Here's how the part is built. I have some questions about the finished solid (model axes, mm). Round coordinates to 2 decimals unless told otherwise and drop trailing zeros. Write each loop counter-clockwise with the first axis right and the second up, starting at its lowest first coordinate (ties: lowest second). Pieces come first, ordered by that corner, then holes. Notation, with made-up numbers: (6, 43) -> (40, 43) arc R33 cw to (40, 80) -> close; hole circle Ø11 at (47.5, 9). An arc over 180 degrees is marked (long way). Put each result on its own line as item: value. Start each with the question number.
1) I want a section at A-A, the plane x = 6. List the corners of the cut face in (y, z) for me, then the cut area to 3 significant figures.
2) I want a section at B-B, the plane z = 8. List the corners of the cut face in (x, y) for me, then the cut area to 3 significant figures.
3) If I drill on line 1 along Z through (x, y) = (4.25, -94.5); line 2 along X through (y, z) = (-51.5, 18.5); line 3 along X through (y, z) = (-12.5, 24), over which ranges is the centre line in solid material (lowest first)? Write a range as [from, to].
4) Will these pins go through, and if not, where does the flat tip stop? P1, Ø5, axis at y = -19, z = 30, coming from the +X side; P2, Ø2.5, axis at x = 4, y = -53.5, coming from the +Z side; P3, Ø11, axis at y = -14, z = 20, coming from the +X side.
5) We'd pull the mould along Y, two halves only. Please class faces 1 (the flat face through (2, -12, 35.029)), 2 (the cylindrical face through (5.2, -16.61, 23.31)), 3 (the cylindrical face through (5.2, -118.17, 20.19)), 4 (the flat face through (2, -127, 10)): released by +Y, released by -Y, zero draft, split by the parting line, or undercut.
from build123d import *

# Parameters (mm, degrees)
F1_DEPTH = 127
F2_R     = 4.4102581717
F2_R_2   = 4.8994098274
F3_DEPTH = 4.5
F5_DEPTH = 25


with BuildPart() as f1:
    # F0 (on Front) → F1 (new body)
    with BuildSketch(Plane.XZ):
        Polygon((0, 35.0287221372), (0, 0), (7.501238957, 0), (7.501238957, 2.9951336328), (2.985865809, 2.9951336328), (2.985865809, 35.0287221372), align=None)
    extrude(amount=F1_DEPTH)

    # F2 (on face) → F3 (join)
    with BuildSketch(Plane.YZ.offset(2.985865809)):
        with Locations((-113.7654781342, 19.9951336328)):
            Circle(F2_R)
        with Locations((-13, 19.9951336328)):
            Circle(F2_R_2)
    extrude(amount=F3_DEPTH)

    # F4 (on face) → F5 (cut)
    with BuildSketch(Plane.YZ.offset(2.985865809)):
        with BuildLine():
            Line((-13.2493425337, 35.0287221372), (-111.2344633553, 35.0287221372))
            add(Edge.make_bspline(
                [(-111.2344633553, 35.0287221372), (-100.3129034646, 34.2859826119), (-64.8860498538, 4.0545608595), (-24.5372166276, 33.6567649219), (-13.2493425337, 35.0287221372)],
                knots=[0.2100734241, 0.2100734241, 0.2100734241, 0.2100734241, 0.5001806892, 0.7879158408, 0.7879158408, 0.7879158408, 0.7879158408], degree=3))
        make_face()
        with BuildLine():
            Line((-127, 35.0287221372), (-127, 19.011927885))
            add(Edge.make_bspline(
                [(-127, 19.011927885), (-123.3541108211, 26.7616729413), (-119.7082216422, 34.5114179975), (-112.8133311868, 35.0287221372)],
                knots=[0, 0, 0, 0, 0.1956359691, 0.1956359691, 0.1956359691, 0.1956359691], degree=3))
            Line((-112.8133311868, 35.0287221372), (-127, 35.0287221372))
        make_face()
        with BuildLine():
            add(Edge.make_bspline(
                [(-10.2470470592, 35.0287221372), (-4.1562861309, 34.0936794049), (-2.0781430654, 26.552803645), (0, 19.011927885)],
                knots=[0.8155753696, 0.8155753696, 0.8155753696, 0.8155753696, 1, 1, 1, 1], degree=3))
            Line((0, 19.011927885), (0, 35.0287221372))
            Line((0, 35.0287221372), (-10.2470470592, 35.0287221372))
        make_face()
    extrude(amount=-F5_DEPTH, mode=Mode.SUBTRACT)


solid = f1.part
Findings:
1. outline: (-127, 0) -> (0, 0) -> (0, 3) -> (-127, 3) -> close; circle Ø8.82 at (-113.77, 20); circle Ø9.8 at (-13, 20)
1. area: 517 mm2
2. outline: (0, -127) -> (2.99, -127) -> (2.99, 0) -> (0, 0) -> close
2. area: 379 mm2
3. line 1: z = [0, 3]
3. line 2: x = [0, 2.99]
3. line 3: x = [0, 7.49]
4. P1: stops at x = 2.99
4. P2: stops at z = 20.35
4. P3: stops at x = 7.49
5. face 1: zero draft
5. face 2: undercut
5. face 3: undercut
5. face 4: released by -Y
